from build123d import *

# Parameters (mm, degrees)
F0_R     = 38.1
F1_DEPTH = 12.7
F2_R     = 3.81
F3_SIZE  = 7.62
F4_R     = 27.94
F5_DEPTH = 76.2


with BuildPart() as f1:
    # F0 (on Top) → F1 (new body)
    with BuildSketch(Plane.XY):
        Circle(F0_R)
    extrude(amount=F1_DEPTH)

    # F2
    f2_edges = [f1.edges().sort_by_distance(p)[0] for p in [
        (-38.1, 0, 12.7),
    ]]
    fillet(f2_edges, radius=F2_R)

    # F3
    f3_edges = [f1.edges().sort_by_distance(p)[0] for p in [
        (-38.1, 0, 0),
    ]]
    chamfer(f3_edges, length=F3_SIZE)

    # F4 (on face) → F5 (join)
    with BuildSketch(Plane.XY.offset(12.7)):
        Circle(F4_R)
    extrude(amount=F5_DEPTH)


solid = f1.part
CAD build for the part. Positions are in the model's coordinates, mm. A direction names the side the tool comes from. Coordinates: 2 decimals unless noted, no trailing zeros. Write each loop counter-clockwise with the first axis right and the second up, starting at its lowest first coordinate (ties: lowest second). Pieces come first, ordered by that corner, then holes. Notation, with made-up numbers: M 82.25,30 L 136.25,30 A25 cw 136.25,44 Z; hole C 80,57.25 d8. An arc over 180 degrees is marked long. Answer as a JSON object with one key per item and string values. Group by question number.
1) Tool access for faces 1 (the face through (-3.64, 27.7, 50.27)), 2 (the face through (0, 0, 88.9)): list every direction of +Z, -Z, +X, -X, +Y, -Y with a clear straight run to the whole face (end or side of a thin tool).
2) Saw through at D-D (z = 6.5). Write the cut outline in (x, y).
3) Pin check, flat tips, straight feed: pin 1 Ø10 at (y, z) = (-2, 20) entering from +X; pin 2 Ø6 at (x, y) = (5.5, 21) entering from -Z; pin 3 Ø1.5 at (x, z) = (-22.5, 80) entering from +Y; pin 4 Ø8 at (y, z) = (-25.5, 61) entering from +X. Stop position of each tip, or through.
4) Saw through at A-A (x = 0). Write the cut outline in (y, z), plus the area to 3 significant figures.
5) Wall check: line 1 (Z direction, x = -25.5, y = -13); line 2 (X direction, y = -1, z = 78.5); line 3 (Z direction, x = 11.5, y = -33.5). Give the ranges that are in metal, low to high. Write a range as from..to.
6) Saw through at C-C (z = 66). Write the cut outline in (x, y), plus the area to 3 significant figures.
Values follow:
{
 "1": {"face 1": "+Z", "face 2": "+Z, +X, -X, +Y, -Y"},
 "2": {"outline": "C 0,0 d73.96"},
 "3": {"pin 1": "stops at x = 27.94", "pin 2": "stops at z = 0", "pin 3": "stops at y = 17.54", "pin 4": "stops at x = 17.84"},
 "4": {"outline": "M -38.1,7.62 L -30.48,0 L 30.48,0 L 38.1,7.62 L 38.1,8.89 A3.81 ccw 34.29,12.7 L 27.94,12.7 L 27.94,88.9 L -27.94,88.9 L -27.94,12.7 L -34.29,12.7 A3.81 ccw -38.1,8.89 Z", "area": "5,160 mm2"},
 "5": {"line 1": "z = 0..12.7", "line 2": "x = -27.92..27.92", "line 3": "z = 4.94..12.53"},
 "6": {"outline": "C 0,0 d55.88", "area": "2,450 mm2"}
}
